Geometry check sheet. Reference: the model listing, model coordinates, mm. Face numbers are marked on the shaded views. A direction names the side the tool comes from. Round coordinates to 2 decimals unless told otherwise and drop trailing zeros. Order: outer loops, then holes, each group sorted by start corner. A loop starts at its lowest first (then second) coordinate and runs counter-clockwise, first axis right, second up.
(1) Gauge pin test, flat ends, axial feed: P1, Ø4, axis at y = 8.5, z = 5, coming from the -X side; P2, Ø2, axis at y = 11.5, z = 2, coming from the -X side; P3, Ø1, axis at y = 55.5, z = 1.5, coming from the +X side. Record the tip position at first contact, or that the pin passes through.
(2) Cross-section at B-B on z = 4. Enter the section's corners in (x, y).
(3) Cross-section at D-D on x = 36. Enter the section's corners in (y, z), and give its area (3 significant figures).
(4) Cross-section at A-A on y = 41. Enter the section's corners in (x, z), and give its area (4 significant figures).
(5) Draft check along X on the marked faces 1, 2 and 3. Enter one of: pulls with the +X half, pulls with the -X half, needs draft (parallel to the pull), parting line crosses it, or undercut.
(6) Thickness scan on L1, parallel to X at y = 6, z = 5.75; L2, parallel to Y at x = 56, z = 0.75; L3, parallel to X at y = 57, z = 6.5. Record the ranges inside material, lowest first.
(7) Set-up check for the marked faces 4, 5 and 6: record each of +Z, -Z, +X, -X, +Y, -Y from which the full face is reachable in a straight line by a thin tool's end or side.
(8) Cross-section at C-C on x = 55.5. Enter the section's corners in (y, z), and give its area (3 significant figures).
from build123d import *

# Parameters (mm, degrees)
BOSS_EXTRUDE1_DEPTH = 10
FILLET1_R           = 5
CUT_EXTRUDE1_DEPTH  = 10


with BuildPart() as part:
    # Sketch1 → Boss-Extrude1 (new body)
    with BuildSketch(Plane.XY):
        Polygon((0, 0), (15, 0), (15, 10), (30, 80), (45, 10), (45, 0), (60, 0), (60, 5), (50, 5), (50, 10), (30, 103.333333333), (10, 10), (10, 5), (0, 5), align=None)
    extrude(amount=BOSS_EXTRUDE1_DEPTH)

    # Fillet1
    fillet1_edges = [part.edges().sort_by_distance(p)[0] for p in [
        (30, 80, 5),
    ]]
    fillet(fillet1_edges, radius=FILLET1_R)

    # Sketch2 → Cut-Extrude1 (cut)
    with BuildSketch(Plane.XY.offset(10)):
        Polygon((17.180108491, 70), (46.95074544, 70), (40.829828982, 121.012949043), (-8.691955578, 121.012949043), align=None)
    extrude(amount=-CUT_EXTRUDE1_DEPTH, mode=Mode.SUBTRACT)


solid = part.part
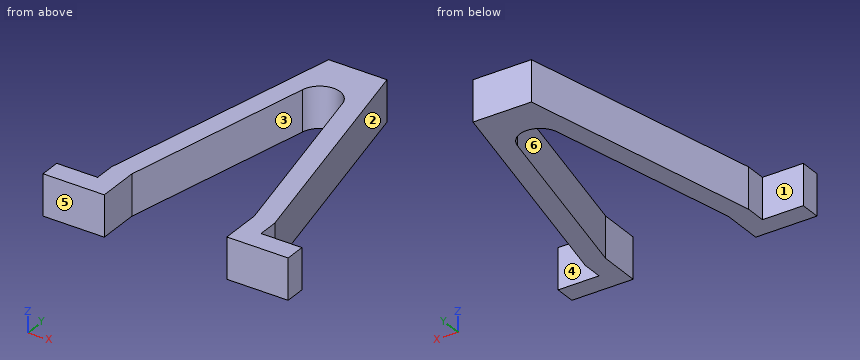
Found:
1. P1: stops at x = 10
1. P2: stops at x = 10.11
1. P3: stops at x = 40.36
2. outline: (0, 0) - (15, 0) - (15, 10) - (25.11, 57.18) arc R5 cw to (34.89, 57.18) - (45, 10) - (45, 0) - (60, 0) - (60, 5) - (50, 5) - (50, 10) - (37.14, 70) - (22.86, 70) - (10, 10) - (10, 5) - (0, 5) - close
3. outline: (52, 0) - (70, 0) - (70, 10) - (52, 10) - close
3. area: 180 mm2
4. outline: (16.64, 0) - (21.64, 0) - (21.64, 10) - (16.64, 10) - close; (38.36, 0) - (43.36, 0) - (43.36, 10) - (38.36, 10) - close
4. area: 100.0 mm2
5. face 1: needs draft
5. face 2: pulls with the +X half
5. face 3: undercut
6. L1: x = 10 to 15, 45 to 50
6. L2: y = 0 to 5
6. L3: x = 20.07 to 25.07, 34.93 to 39.93
7. face 4: +Z, -Z, +X, +Y
7. face 5: +Z, -Z, +X, -X, -Y
7. face 6: +Z, -Z, -Y
8. outline: (0, 0) - (5, 0) - (5, 10) - (0, 10) - close
8. area: 50.0 mm2
